Check sheet for the modelled part. Datum: model origin and axes. Units: mm. A direction names the side the tool comes from. Round coordinates to 2 decimals unless told otherwise and drop trailing zeros. Order: outer loops, then holes, each group sorted by start corner. A loop starts at its lowest first (then second) coordinate and runs counter-clockwise, first axis right, second up. Notation, with made-up numbers: (-33, 63.5) -> (3, 63.5) arc R19 ccw to (3, 73.5) -> close; hole circle Ø6 at (69, 77). An arc over 180 degrees is marked (long way). Answer in a Markdown table with one row per item. Add a question column.
1. Depth check by flat-ended pin: P1, Ø10, axis at x = 39.5, y = -0.5, coming from the -Z side; P2, Ø1, axis at y = -14, z = -4, coming from the -X side; P3, Ø9, axis at x = 21, z = 4.5, coming from the -Y side; P4, Ø0.8, axis at y = 11.5, z = 2, coming from the -X side. Enter the tip coordinate at first touch or a pass-through.
2. Material ranges on L1, parallel to Y at x = 20, z = 6.75; L2, parallel to Y at x = -18, z = 4; L3, parallel to Y at x = 32, z = 3.5, recorded low to high. Write a range as from..to.
3. Draft check along Z on faces 5 (the flat face through (-2, 1.268, 0)), 6 (the flat face through (-14, 0, -3.5)), 7 (the flat face through (21.884, 23, 0)), 8 (the flat face through (21.884, 18, -6)). Enter one of: +Z half, -Z half, draft (parallel to the pull), parting line (faces both ways), or undercut.
4. Sectioned sample at C-C, the plane y = -15. Record the boundary of the cut face in (x, z), then the cut area to 3 significant figures.
5. Sectioned sample at B-B, the plane z = -6.75. Count the separate pieces of the cut face and the enclosed holes in it, then the cut area to 3 significant figures.
6. Sectioned sample at D-D, the plane y = -26. Record the boundary of the cut face in (x, z).
7. Sectioned sample at A-A, the plane x = 3.5. Record the boundary of the cut face in (y, z), then the cut area to 3 significant figures.
8. Access from +Z, -Z, +X, -X, +Y, -Y to the whole of each face (thin tool, end or side, straight path). Record for faces 1 (the flat face through (-4, -10.732, 0)), 2 (the flat face through (52, 13.168, 0)), 3 (the flat face through (-20, 6.268, -6)), 4 (the flat face through (31.053, 25, 0)).
```python
from build123d import *

# Parameters (mm, degrees)
F1_DEPTH  = 9.5
F3_DEPTH  = 18
F4_R      = 4.5
F5_DEPTH  = 40
F6_W      = 10.7216464161
F6_H      = 8
F7_DEPTH  = 2
F8_R      = 1
F9_DEPTH  = 5
F8_W      = 1
F8_H      = 3
F10_DEPTH = 18
F11_DEPTH = 18
F12_R     = 1
F13_DEPTH = 6.9
F15_DEPTH = 3
F16_R     = 1.25
F17_DEPTH = 5
F18_DEPTH = 25


with BuildPart() as f1:
    # F0 (on Top) → F1 (new body, symmetric)
    with BuildSketch(Plane.XY):
        Polygon((60.1971853051, 26.2679918303), (-39.8028146949, 26.2679918303), (-44.8028146949, 6.2679918303), (-24.8028146949, 6.2679918303), (-31.8558939232, -33.7320081697), (-6.8558939232, -33.7320081697), (0.1971853051, 6.2679918303), (60.1971853051, 6.2679918303), align=None)
    extrude(amount=F1_DEPTH, both=True)

    # F2 (on face) → F3 (cut)
    with BuildSketch(Plane.XY.offset(9.5)):
        Polygon((21.8837381179, 24.7679918303), (-38.1162618821, 24.7679918303), (-42.2412618821, 8.2679918303), (-22.4193075097, 8.2679918303), (-27.2986237894, -19.4039858791), (-6.3603302369, -19.4039858791), (-1.8336679186, 6.2679918303), (-17.4193075097, 6.2679918303), (-17.4193075097, 8.2679918303), (56.8837381179, 8.2679918303), (56.8837381179, 11.2679918303), (21.8837381179, 11.2679918303), align=None)
    extrude(amount=-F3_DEPTH, mode=Mode.SUBTRACT)

    # F4 (on face) → F5 (cut)
    with BuildSketch(Plane.YZ.offset(60.1971853051)):
        with Locations((19.7679918303, 0)):
            Circle(F4_R)
    extrude(amount=-F5_DEPTH, mode=Mode.SUBTRACT)

    # F6 (on Top) → F7 (cut, symmetric)
    with BuildSketch(Plane.XY):
        Polygon((31.0530696271, 22.4650362791), (31.0530696271, 31.3576222958), (-16.5646290837, 30.772159468), (-16.5646290837, 22.4650362791), align=None)
        with Locations((-41.1441657065, 17.2679918303)):
            Rectangle(F6_W, F6_H)
    extrude(amount=F7_DEPTH, both=True, mode=Mode.SUBTRACT)

    # F8 (on face) → F9 (join)
    with BuildSketch(Plane.XY.offset(-8.5)):
        Polygon((-41.4912618821, 11.2679918303), (21.8837381179, 11.2679918303), (21.8837381179, 12.2679918303), (20.8837381179, 12.2679918303), (-41.2412618821, 12.2679918303), align=None)
        Polygon((-17.4193075097, 6.2679918303), (-22.7719614711, 6.2679918303), (-24.8589656495, -5.5679970244), (-3.9206720971, -5.5679970244), (-1.8336679186, 6.2679918303), align=None)
        Polygon((-28.4193075097, 14.2679918303), (-24.4193075097, 14.2679918303), (-22.2943075097, 22.7679918303), (-26.2943075097, 22.7679918303), align=None)
        with Locations((-25.3568075097, 18.5179918303)):
            Circle(F8_R, mode=Mode.SUBTRACT)
    extrude(amount=F9_DEPTH)

    # F8 (on face) → F10 (join, through all)
    with BuildSketch(Plane.XY.offset(-8.5)):
        with Locations((21.3837381179, 23.2679918303)):
            Rectangle(F8_W, F8_H)
    extrude(amount=F10_DEPTH)

    # F8 (on face) → F11 (join, through all)
    with BuildSketch(Plane.XY.offset(-8.5)):
        with Locations((21.3837381179, 13.7679918303)):
            Rectangle(F8_W, F8_H)
    extrude(amount=F11_DEPTH)

    # F12 (on face) → F13 (cut)
    with BuildSketch(Plane.XZ.offset(-6.2679918303)):
        with Locations((52.1971853051, 0)):
            Circle(F12_R)
    extrude(amount=-F13_DEPTH, mode=Mode.SUBTRACT)

    # F14 (on Top) → F15 (cut, symmetric)
    with BuildSketch(Plane.XY):
        Polygon((7.0393216934, 1.2679918303), (-9.7211528242, 1.2679918303), (-8.9475925263, -10.7320081697), (7.0393216934, -10.7320081697), align=None)
    extrude(amount=F15_DEPTH, both=True, mode=Mode.SUBTRACT)

    # F16 (on face) → F17 (cut)
    with BuildSketch(Plane.XY.offset(-8.5)):
        with Locations((-7.9571865499, 1.7126952298)):
            Circle(F16_R)
    extrude(amount=-F17_DEPTH, mode=Mode.SUBTRACT)

    # F18 (cut): a face of the model
    f18_faces = [f1.faces().sort_by_distance(p)[0] for p in [
        (-7.9571865499, 1.7126952298, -8.5),
    ]]
    extrude(f18_faces, amount=-F18_DEPTH, mode=Mode.SUBTRACT)


solid = f1.part
```
Answer key:
| question | item | result |
|---|---|---|
| 1 | P1 | passes through |
| 1 | P2 | stops at x = -28.46 |
| 1 | P3 | stops at y = 6.27 |
| 1 | P4 | stops at x = -43.59 |
| 2 | L1 | y = 6.27..8.27, 24.77..26.27 |
| 2 | L2 | y = -33.73..-19.4, 24.77..26.27 |
| 2 | L3 | y = 6.27..8.27, 11.27..16.94, 22.6..26.27 |
| 3 | face 5 | undercut |
| 3 | face 6 | +Z half |
| 3 | face 7 | undercut |
| 3 | face 8 | draft |
| 4 | outline | (-28.55, -9.5) -> (-3.55, -9.5) -> (-3.55, 9.5) -> (-5.58, 9.5) -> (-5.58, -8.5) -> (-26.52, -8.5) -> (-26.52, 9.5) -> (-28.55, 9.5) -> close |
| 4 | area | 98.1 mm² |
| 5 | separate pieces | 2 |
| 5 | enclosed holes | 5 |
| 5 | area | 1,720 mm² |
| 6 | outline | (-30.49, -9.5) -> (-5.49, -9.5) -> (-5.49, 9.5) -> (-30.49, 9.5) -> close |
| 7 | outline | (6.27, -9.5) -> (26.27, -9.5) -> (26.27, -2) -> (24.77, -2) -> (24.77, -8.5) -> (12.27, -8.5) -> (12.27, -3.5) -> (11.27, -3.5) -> (11.27, -8.5) -> (8.27, -8.5) -> (8.27, 9.5) -> (6.27, 9.5) -> close; (24.77, 2) -> (26.27, 2) -> (26.27, 9.5) -> (24.77, 9.5) -> close |
| 7 | area | 82.0 mm² |
| 8 | face 1 | +X |
| 8 | face 2 | -Y |
| 8 | face 3 | +Z |
| 8 | face 4 | +Y |
